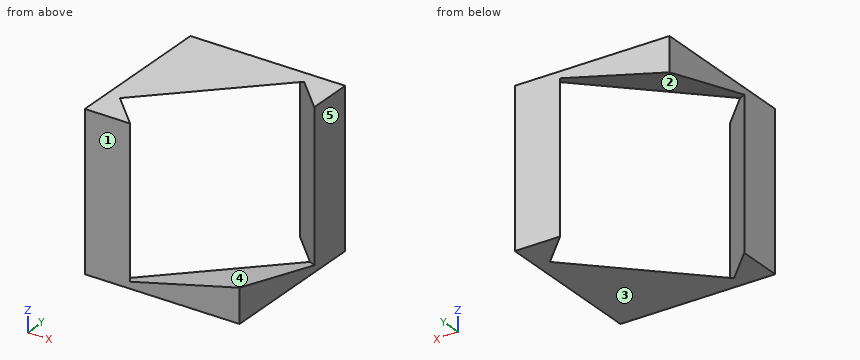
```python
from build123d import *

# Parameters (mm, degrees)
F0_W          = 10
F0_H          = 10
F1_DEPTH      = 10
F6_DEPTH      = 8.334333
F6_DEPTH_BACK = 8.334333


with BuildPart() as f1:
    # F0 (on Top) → F1 (new body)
    with BuildSketch(Plane.XY):
        Rectangle(F0_W, F0_H)
    extrude(amount=F1_DEPTH)

    # F5 (on face) → F6 (cut, two sides)
    with BuildSketch(Plane(origin=(1.111111, -1.111111, 0.555556), x_dir=(-0.745356, -0.596285, 0.298142), z_dir=(-0.666667, 0.666667, -0.333333))) as f6_sk:
        Polygon((-4.833843, 1.309858), (4.65299, -1.852419), (7.815267, 7.634414), (-1.671566, 10.796691), align=None)
    extrude(amount=F6_DEPTH, mode=Mode.SUBTRACT)
    extrude(f6_sk.sketch, amount=-F6_DEPTH_BACK, mode=Mode.SUBTRACT)


solid = f1.part
```
Verification items for the finished model (mm, model axes). Face numbers are marked on the shaded views. A direction names the side the tool comes from. Round coordinates to 2 decimals unless told otherwise and drop trailing zeros. Write each loop counter-clockwise with the first axis right and the second up, starting at its lowest first coordinate (ties: lowest second). Pieces come first, ordered by that corner, then holes. Notation, with made-up numbers: (35.5, 0.25) -> (67.5, 0.25) arc R27 ccw to (67.5, 31.25) -> close; hole circle Ø10 at (41, 30). An arc over 180 degrees is marked (long way). Write each question's results on one line, items separated by ' | '.
Q1. Sectioned sample at C-C, the plane z = 2. Record the boundary of the cut face in (x, y).
Derived:
outline: (-5, -5) -> (-2.07, -5) -> (-5, -2.07) -> close; (2.07, 5) -> (5, 2.07) -> (5, 5) -> close; (4.21, -5) -> (5, -5) -> (5, -4.21) -> close
Q2. Sectioned sample at D-D, the plane z = 1. Record the boundary of the cut face in (x, y), and give its area (3 significant figures).
Derived:
outline: (-5, -5) -> (-2.07, -5) -> (-5, -2.07) -> close; (0.21, -5) -> (5, -5) -> (5, -0.21) -> close; (2.07, 5) -> (5, 2.07) -> (5, 5) -> close | area: 20.0 mm²
Q3. Sectioned sample at B-B, the plane x = 1.75. Record the boundary of the cut face in (y, z).
Derived:
outline: (-5, 0) -> (0.54, 0) -> (-5, 1.38) -> close; (2.96, 10) -> (5, 9.49) -> (5, 10) -> close
Q4. Access from +Z, -Z, +X, -X, +Y, -Y to the whole of each face (thin tool, end or side, straight path). Record for the marked faces 4 and 5.
Derived:
face 4: +Z | face 5: +Z, -Z, +X, +Y, -Y
Q5. Sectioned sample at A-A, the plane z = 5.5. Record the boundary of the cut face in (x, y).
Derived:
outline: (-5, -5) -> (-2.07, -5) -> (-5, -2.07) -> close; (2.07, 5) -> (5, 2.07) -> (5, 5) -> close
Q6. Go/stop test with a flat-tipped pin: pin 1 Ø1 at (y, z) = (-3, 8) entering from +X. Record where the tip stops, or that it passes through.
Derived:
pin 1: stops at x = -3.57
Q7. Draft check along Y on the marked faces 1, 2 and 3. Enter one of: released by +Y, released by -Y, zero draft, split by the parting line, or undercut.
Derived:
face 1: released by -Y | face 2: undercut | face 3: zero draft
Q8. Thickness scan on probe 1 along Y at (x, z) = (-3.5, 5); probe 2 along Z at (x, y) = (2.5, 0); probe 3 along X at (y, z) = (-2.75, 6.75). Record the ranges inside material, lowest first.
Derived:
probe 1: y = -5 to -3.57 | probe 2: z = 0 to 0.32 | probe 3: x = -5 to -4.32
